The figure shows three views and two pictorial views of one solid part (mm, origin at its lowest corner). Answer the questions. A direction names the side the tool comes from. Give positions to 0.01 mm unless a question says otherwise; leave off trailing zeros. Loops run counter-clockwise (first coordinate to the right, second up) from the corner with the lowest first, then second, coordinate; pieces in that order, holes last. Notation, with made-up numbers: (20.25, -36) - (48.25, -36) arc R13 ccw to (48.25, -24) - close; hole circle Ø3 at (84.5, 23). An arc over 180 degrees is marked (long way). Use CSV: the item, a comma, the result in double quotes.
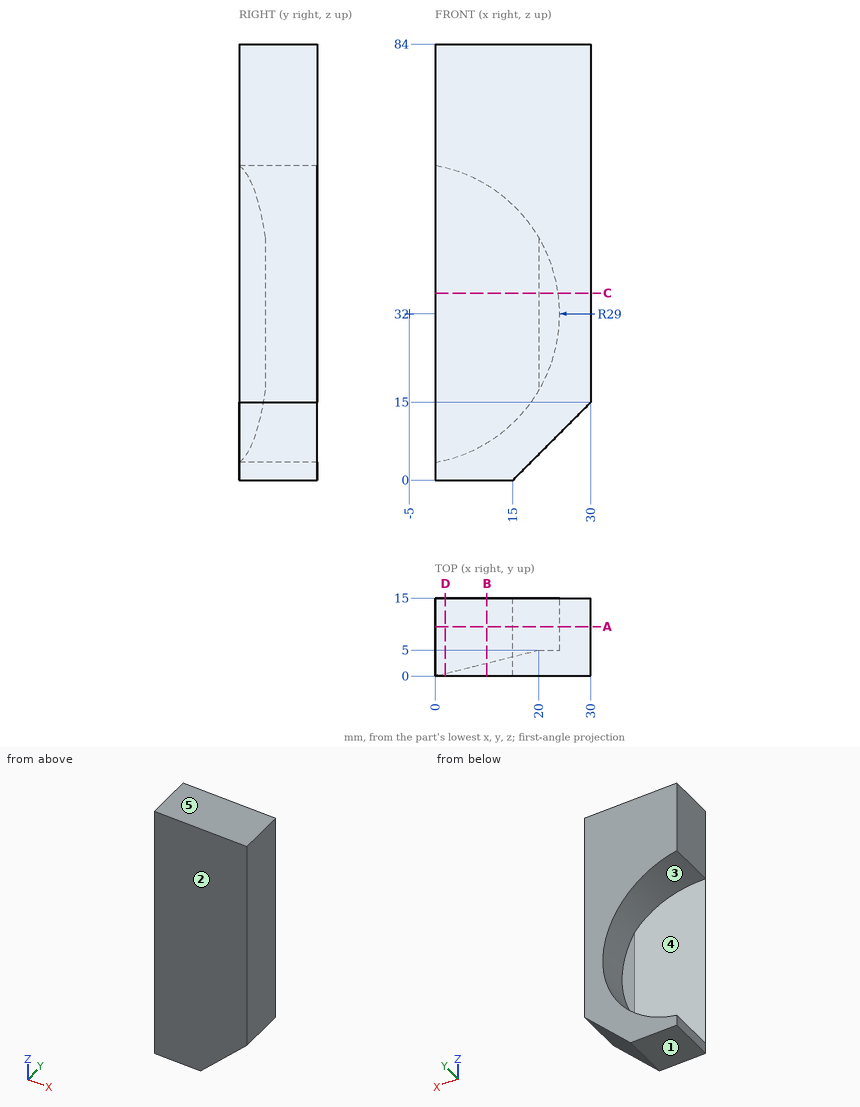
Item 1: The mould has two halves that part along Z. Classify the marked faces 1, 2 and 3: pulls with the +Z half, pulls with the -Z half, needs draft (parallel to the pull), parting line crosses it, or undercut.
Determined:
face 1,"pulls with the -Z half"
face 2,"needs draft"
face 3,"undercut"
Item 2: Find the intervals of material crossed by line 1 (Z direction, x = 8.5, y = 7.5); line 2 (Z direction, x = 10.5, y = 13.25); line 3 (X direction, y = 6.5, z = 7.5), in increasing order.
Determined:
line 1,"z = 0 to 6.33, 57.67 to 84"
line 2,"z = 0 to 7.49, 56.51 to 84"
line 3,"x = 10.52 to 22.5"
Item 3: For the marked faces 4 and 5, determine the directions among +Z, -Z, +X, -X, +Y, -Y from which every point of the face is accessible in a straight line to the end or side of a thin tool.
Determined:
face 4,"-X, +Y"
face 5,"+Z, +X, -X, +Y, -Y"
Item 4: A cutting plane is placed at D-D on x = 2. Determine the outline of the cut face in (y, z), and give its area (3 significant figures).
Determined:
outline,"(0, 0) - (15, 0) - (15, 3.86) - (0.5, 3.86) - (0.5, 60.14) - (15, 60.14) - (15, 84) - (0, 84) - close"
area,"444 mm²"
Item 5: A cutting plane is placed at A-A on y = 9.5. Determine the outline of the cut face in (x, z).
Determined:
outline,"(0, 0) - (15, 0) - (30, 15) - (30, 84) - (0, 84) - (0, 60.57) arc R29 cw to (0, 3.43) - close"
Item 6: A cutting plane is placed at C-C on z = 36. Determine the outline of the cut face in (x, y).
Determined:
outline,"(0, 0) - (30, 0) - (30, 15) - (23.72, 15) - (23.72, 5) - (20, 5) - close"
Item 7: A cutting plane is placed at B-B on x = 10. Determine the outline of the cut face in (y, z).
Determined:
outline,"(0, 0) - (15, 0) - (15, 7.18) - (2.5, 7.18) - (2.5, 56.82) - (15, 56.82) - (15, 84) - (0, 84) - close"
